Input: part model. Units: mm. Frame: model coordinates. A direction names the side the tool comes from. Coordinates: 2 decimals unless noted, no trailing zeros. Loops run counter-clockwise (first coordinate to the right, second up) from the corner with the lowest first, then second, coordinate; pieces in that order, holes last. Notation, with made-up numbers: M 25,1 L 39,1 A16 cw 39,10 Z; hole C 34,36.5 d1. An arc over 180 degrees is marked long. Use a Markdown table: item, result. Add a question column.
1. Section B-B on y = -7. Output: boundary loops of the cut face in (x, z), then the cut area to 3 significant figures.
2. Draft query along Y for faces 5 (the cylindrical face through (0, -16, 1)), 6 (the cylindrical face through (11, 2, 1)), 7 (the cylindrical face through (11, -15, 1)). Return one class per face: +Y half, -Y half, draft (parallel to the pull), parting line (faces both ways), or undercut.
3. Section C-C on x = 0. Output: boundary loops of the cut face in (y, z), then the cut area to 3 significant figures.
4. Line query: L1, parallel to Y at x = 11, z = 2; L2, parallel to X at y = -0.5, z = 2.45; L3, parallel to Y at x = 4, z = 5.55. Output: solid intervals per line, ascending. Write a range as [from, to].
5. Section D-D on y = 0. Output: boundary loops of the cut face in (x, z).
6. Set-up query: faces 1 (the cylindrical face through (-0.3, -7.1, 4.5)), 2 (the flat face through (5, -13, 1)), 3 (the flat face through (5, -3.5, 4)), 4 (the flat face through (6, -1, 1)). Return all of +Z, -Z, +X, -X, +Y, -Y with unobstructed straight access to the full face (end or side cutting, diameter ignored); none if empty.
7. Section A-A on z = 1.4. Output: boundary loops of the cut face in (x, y).
8. Pin query (flat end, axial travel): pin 1 (2.5 mm diameter, centred on x = 5.5, z = 4.5, fed in from +Y); pin 2 (2.5 mm diameter, centred on x = 11, y = -14, fed in from +Z); pin 3 (1.5 mm diameter, centred on x = 5, z = 4.5, fed in from -Y). Return the tip coordinate at first contact, or that it passes through.
```python
from build123d import *

# Parameters (mm, degrees)
SKETCH_1_R      = 1
EXTRUDE_1_DEPTH = 3
EXTRUDE_2_DEPTH = 3


with BuildPart() as part:
    # 草图1 → 凸台-拉伸1 (new body)
    with BuildSketch(Plane.XY):
        with BuildLine():
            Line((3, -13), (8, -13))
            ThreePointArc((8, -13), (11, -16), (14, -13))
            Line((14, -13), (14, -1))
            ThreePointArc((14, -1), (11, 2), (8, -1))
            Line((8, -1), (3, -1))
            ThreePointArc((3, -1), (0, 2), (-3, -1))
            Line((-3, -1), (-3, -13))
            ThreePointArc((-3, -13), (0, -16), (3, -13))
        make_face()
        with Locations((11, -14)):
            Circle(SKETCH_1_R, mode=Mode.SUBTRACT)
        Circle(SKETCH_1_R, mode=Mode.SUBTRACT)
        with Locations((11, 0)):
            Circle(SKETCH_1_R, mode=Mode.SUBTRACT)
        with Locations((0, -14)):
            Circle(SKETCH_1_R, mode=Mode.SUBTRACT)
    extrude(amount=EXTRUDE_1_DEPTH)

    # 草图2 → 凸台-拉伸2 (add)
    with BuildSketch(Plane.XY.offset(3)):
        with BuildLine():
            Line((3.2, -3.5), (7.8, -3.5))
            ThreePointArc((7.8, -3.5), (11.3, -7), (7.8, -10.5))
            Line((7.8, -10.5), (3.2, -10.5))
            ThreePointArc((3.2, -10.5), (-0.3, -7), (3.2, -3.5))
        make_face()
    extrude(amount=EXTRUDE_2_DEPTH)


solid = part.part
```
Answers below:
| question | item | result |
|---|---|---|
| 1 | outline | M -3,0 L 14,0 L 14,3 L 11.3,3 L 11.3,6 L -0.3,6 L -0.3,3 L -3,3 Z |
| 1 | area | 85.8 mm² |
| 2 | face 5 | -Y half |
| 2 | face 6 | +Y half |
| 2 | face 7 | undercut |
| 3 | outline | M -16,0 L -15,0 L -15,3 L -16,3 Z; M -13,0 L -1,0 L -1,3 L -5.58,3 L -5.58,6 L -8.42,6 L -8.42,3 L -13,3 Z; M 1,0 L 2,0 L 2,3 L 1,3 Z |
| 3 | area | 50.5 mm² |
| 4 | L1 | y = [-16, -15], [-13, -1], [1, 2] |
| 4 | L2 | x = [-2.96, -0.87], [0.87, 2.96], [8.04, 10.13], [11.87, 13.96] |
| 4 | L3 | y = [-10.5, -3.5] |
| 5 | outline | M -2.83,0 L -1,0 L -1,3 L -2.83,3 Z; M 1,0 L 2.83,0 L 2.83,3 L 1,3 Z; M 8.17,0 L 10,0 L 10,3 L 8.17,3 Z; M 12,0 L 13.83,0 L 13.83,3 L 12,3 Z |
| 6 | face 1 | +Z, -X |
| 6 | face 2 | +Z, -Z, -Y |
| 6 | face 3 | +Z, +X, -X, +Y |
| 6 | face 4 | +Z, -Z, +Y |
| 7 | outline | M -3,-13 A3 ccw 3,-13 L 8,-13 A3 ccw 14,-13 L 14,-1 A3 ccw 8,-1 L 3,-1 A3 ccw -3,-1 Z; hole C 0,-14 d2; hole C 0,0 d2; hole C 11,-14 d2; hole C 11,0 d2 |
| 8 | pin 1 | stops at y = -3.5 |
| 8 | pin 2 | stops at z = 3 |
| 8 | pin 3 | stops at y = -10.5 |
